```python
from build123d import *

# Parameters (mm, degrees)
SKETCH1_W                                    = 450
SKETCH1_H                                    = 100
BOSS_EXTRUDE1_DEPTH                          = 10
CBORE_FOR_M4_HEX_HEAD_CAP_SCREW1_D           = 4.5
CBORE_FOR_M4_HEX_HEAD_CAP_SCREW1_CBORE_D     = 11.083
CBORE_FOR_M4_HEX_HEAD_CAP_SCREW1_CBORE_DEPTH = 2.8
M5_TAPPED_HOLE1_D                            = 4.2


with BuildPart() as part:
    # Sketch1 → Boss-Extrude1 (new body)
    with BuildSketch(Plane(origin=(0, 0, 0), x_dir=(1, 0, 0), z_dir=(0, 1, 0))):
        Rectangle(SKETCH1_W, SKETCH1_H)
    extrude(amount=BOSS_EXTRUDE1_DEPTH)

    # CBORE for M4 Hex Head Cap Screw1 (through all)
    with Locations(Plane(origin=(0, 10, 0), x_dir=(1, 0, 0), z_dir=(0, 1, 0))):
        with Locations((205, -38), (205, 38), (-35, 38), (-35, -38)):
            CounterBoreHole(CBORE_FOR_M4_HEX_HEAD_CAP_SCREW1_D / 2, CBORE_FOR_M4_HEX_HEAD_CAP_SCREW1_CBORE_D / 2, CBORE_FOR_M4_HEX_HEAD_CAP_SCREW1_CBORE_DEPTH)

    # M5 Tapped Hole1 (through all)
    with Locations(Plane(origin=(0, 10, 0), x_dir=(1, 0, 0), z_dir=(0, 1, 0))):
        with Locations((-50, 26), (-50, -26), (-196, -26), (-196, 26)):
            Hole(M5_TAPPED_HOLE1_D / 2)


solid = part.part
```
Can you work these out from the model? Positions are in its coordinate system, mm. A direction names the side the tool comes from. Round coordinates to 2 decimals unless told otherwise and drop trailing zeros. Answer in a Markdown table with one row per item.
1. On a 3-axis mill with a long thin cutter (end or side, diameter ignored), from which of +Z, -Z, +X, -X, +Y, -Y can I reach the whole of each face in a straight line? I mean faces 4 (the face through (-3, 10, -1)), 5 (the face through (207.4, 7.2, 37.9)). Say none if no direction works.
Established:
| item | result |
|---|---|
| face 4 | +Z, -Z, +X, -X, +Y |
| face 5 | +Y |
2. Thinking about a two-plate mould opening in X: for faces 1 (the face through (-36.2, 8.62, -32.59)), 2 (the face through (-3, 5, 50)), 3 (the face through (225, 5, 1)), which applies, pulls with the +X half, pulls with the -X half, needs draft (parallel to the pull), parting line crosses it, or undercut?
Established:
| item | result |
|---|---|
| face 1 | undercut |
| face 2 | needs draft |
| face 3 | pulls with the +X half |
3. Please list where these lines run through material, in increasing order: line 1 (X direction, y = 8.95, z = 38); line 2 (Z direction, x = -196, y = 5); line 3 (X direction, y = 5.5, z = -38). Write a range as from..to.
Established:
| item | result |
|---|---|
| line 1 | -225..-40.54, -29.46..199.46, 210.54..225 |
| line 2 | -50..-28.1, -23.9..23.9, 28.1..50 |
| line 3 | -225..-37.25, -32.75..202.75, 207.25..225 |
4. I'm going to push a flat-ended pin straight in: pin 1 Ø5.5 at (x, z) = (-36, 37.5) entering from +Y. Where does the tip first touch, or does it pass through?
Established:
| item | result |
|---|---|
| pin 1 | y = 7.2 |
